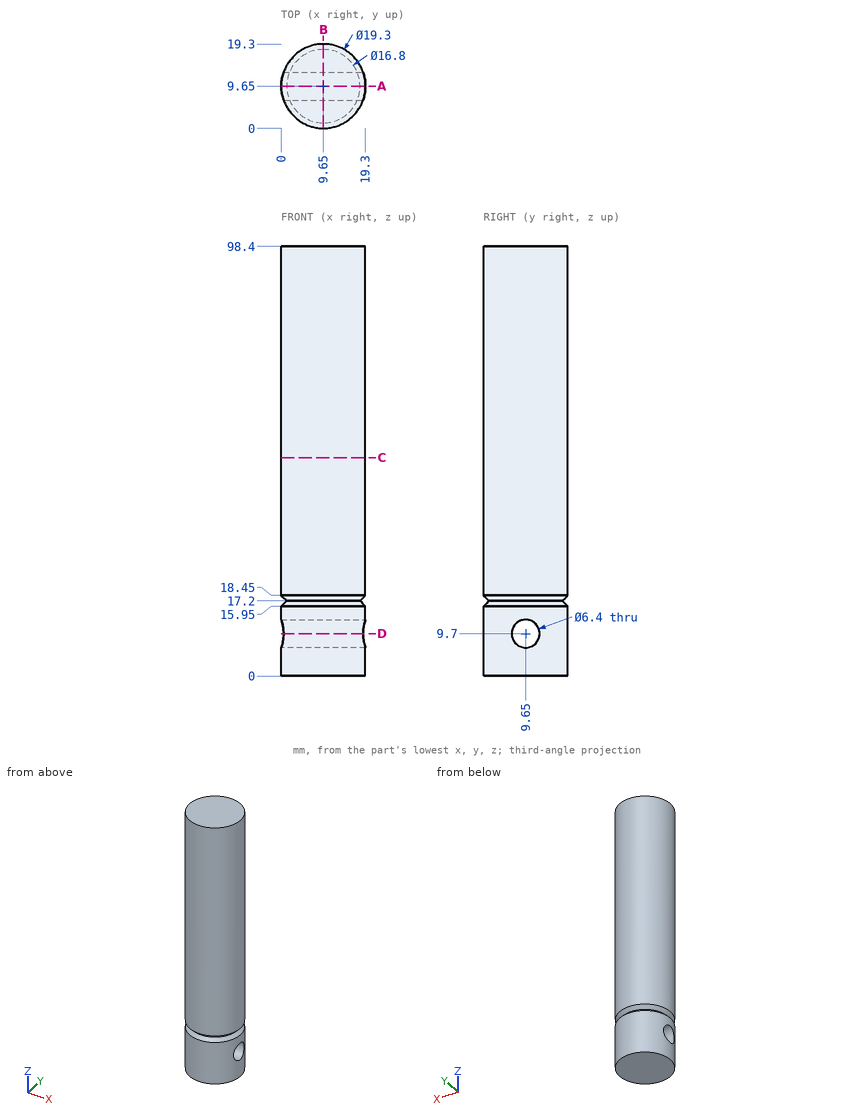
Study the drawing (mm; zero at the part's minimum x, y, z) and answer. Round coordinates to 2 decimals unless told otherwise and drop trailing zeros. Write each loop counter-clockwise with the first axis right and the second up, starting at its lowest first coordinate (ties: lowest second). Pieces come first, ordered by that corner, then holes.
Q1. Straight lines are drawn through the part: line 1 (Z direction, x = 6.5, y = 9.5); line 2 (Z direction, x = 2.25, y = 15.25); line 3 (Y direction, x = 4, z = 9.7). For each, find the intervals that lie inside material, in ascending order.
Values:
line 1: z = 0 to 6.5, 12.9 to 98.4
line 2: z = 0 to 16.32, 18.08 to 98.4
line 3: y = 1.83 to 6.45, 12.85 to 17.47
Q2. Find section C-C on z = 50. Determine the outline of the cut face in (x, y).
Values:
outline: circle Ø19.3 at (9.65, 9.65)
Q3. Find section A-A on y = 9.65. Determine the outline of the cut face in (x, z), and give its area (3 significant figures).
Values:
outline: (0, 0) - (19.3, 0) - (19.3, 6.5) - (0, 6.5) - close; (0, 12.9) - (19.3, 12.9) - (19.3, 15.95) - (18.05, 17.2) - (19.3, 18.45) - (19.3, 98.4) - (0, 98.4) - (0, 18.45) - (1.25, 17.2) - (0, 15.95) - close
area: 1,770 mm2
Q4. Find section D-D on z = 9.7. Determine the outline of the cut face in (x, y), and give its area (3 significant figures).
Values:
outline: (0.55, 6.45) arc R9.65 ccw to (18.75, 6.45) - close; (0.55, 12.85) - (18.75, 12.85) arc R9.65 ccw to start
area: 171 mm2
Q5. Flat-ended cylindrical pins translate along their axes: P1, Ø1.5, axis at y = 17, z = 48, coming from the -X side; P2, Ø6, axis at y = 9.65, z = 9.7, coming from the +X side; P3, Ø1, axis at y = 16, z = 66, coming from the +X side; P4, Ø10, axis at x = 15.5, z = 17.5, coming from the +Y side. Find the tip coordinate at first contact, or state that the pin passes through.
Values:
P1: stops at x = 2.61
P2: passes through
P3: stops at x = 17.32
P4: stops at y = 19.25
Q6. Find section B-B on x = 9.65. Determine the outline of the cut face in (y, z).
Values:
outline: (0, 0) - (19.3, 0) - (19.3, 15.95) - (18.05, 17.2) - (19.3, 18.45) - (19.3, 98.4) - (0, 98.4) - (0, 18.45) - (1.25, 17.2) - (0, 15.95) - close; hole circle Ø6.4 at (9.65, 9.7)
